from build123d import *

# Parameters (mm, degrees)
BOSS_EXTRUDE1_DEPTH  = 3.175
M3_CLEARANCE_HOLE1_D = 3.2
SKETCH4_R            = 2.1336
CUT_EXTRUDE1_DEPTH   = 74.133031325
SKETCH5_W            = 3
SKETCH5_H            = 19.05
CUT_EXTRUDE2_DEPTH   = 74.133031325


with BuildPart() as part:
    # Sketch1 → Boss-Extrude1 (new body)
    with BuildSketch(Plane(origin=(0, 0, 0), x_dir=(1, 0, 0), z_dir=(0, 1, 0))):
        Polygon((0, 0), (19.05, 0), (19.05, -3.175), (38.1, -3.175), (38.1, 0), (51.435, 0), (51.435, 7.62), (46.6725, 7.62), (46.6725, 15.24), (51.435, 15.24), (51.435, 22.86), (46.6725, 22.86), (46.6725, 30.48), (51.435, 30.48), (51.435, 51.8922), (0, 51.8922), align=None)
    extrude(amount=BOSS_EXTRUDE1_DEPTH)

    # M3 Clearance Hole1 (through all)
    with Locations(Plane(origin=(0, 3.175, 0), x_dir=(1, 0, 0), z_dir=(0, 1, 0))):
        with Locations((48.26, 19.05)):
            Hole(M3_CLEARANCE_HOLE1_D / 2)

    # Sketch4 → Cut-Extrude1 (cut, through all)
    with BuildSketch(Plane(origin=(0, 3.175, 0), x_dir=(1, 0, 0), z_dir=(0, 1, 0))):
        with Locations(Location((28.575, 27.305, 0), (0, 0, 270))):
            Circle(SKETCH4_R)
    extrude(amount=-CUT_EXTRUDE1_DEPTH, mode=Mode.SUBTRACT)

    # Sketch5 → Cut-Extrude2 (cut, through all)
    with BuildSketch(Plane(origin=(0, 3.175, 0), x_dir=(1, 0, 0), z_dir=(0, 1, 0))):
        with Locations((4.215, 19.05)):
            Rectangle(SKETCH5_W, SKETCH5_H)
    extrude(amount=-CUT_EXTRUDE2_DEPTH, mode=Mode.SUBTRACT)


solid = part.part
Check sheet for the modelled part. Datum: model origin and axes. Units: mm. A direction names the side the tool comes from. Round coordinates to 2 decimals unless told otherwise and drop trailing zeros. Order: outer loops, then holes, each group sorted by start corner. A loop starts at its lowest first (then second) coordinate and runs counter-clockwise, first axis right, second up.
Q1. Scan lines: L1, parallel to X at y = 1.25, z = -19.05 (3 decimals); L2, parallel to X at y = 1.65, z = -11 (1 decimal); L3, parallel to Z at x = 28.5, y = 1 (3 decimals). Record each from-to range of solid material in increasing order.
Filled sheet:
L1: x = 0 to 2.715, 5.715 to 46.66, 49.86 to 51.435
L2: x = 0 to 2.7, 5.7 to 46.7
L3: z = -51.892 to -29.437, -25.173 to 3.175
Q2. Cross-section at D-D, the plane x = 39.5. Enter the section's corners in (y, z) (3 decimals), plus the area to 3 significant figures.
Filled sheet:
outline: (0, -51.892) - (3.175, -51.892) - (3.175, 0) - (0, 0) - close
area: 165 mm2
Q3. Set-up check for faces 5 (the face through (5.715, 2, -19)), 6 (the face through (49, 2, -15.24)), 7 (the face through (38.1, 2, 2)): record each of +Z, -Z, +X, -X, +Y, -Y from which the full face is reachable in a straight line by a thin tool's end or side.
Filled sheet:
face 5: +Y, -Y
face 6: +X, +Y, -Y
face 7: +Z, +X, +Y, -Y
Q4. Depth check by flat-ended pin: P1, Ø3, axis at x = 12.5, z = -7.5, coming from the -Y side; P2, Ø1, axis at x = 49, y = 1.5, coming from the +Z side; P3, Ø1, axis at y = 2, z = -14.5, coming from the +X side. Enter the tip coordinate at first touch or a pass-through.
Filled sheet:
P1: stops at y = 0
P2: stops at z = 0
P3: stops at x = 46.67
Q5. Cross-section at B-B, the plane x = 48.26. Enter the section's corners in (y, z) (3 decimals).
Filled sheet:
outline: (0, -51.892) - (3.175, -51.892) - (3.175, -30.48) - (0, -30.48) - close; (0, -22.86) - (3.175, -22.86) - (3.175, -20.65) - (0, -20.65) - close; (0, -17.45) - (3.175, -17.45) - (3.175, -15.24) - (0, -15.24) - close; (0, -7.62) - (3.175, -7.62) - (3.175, 0) - (0, 0) - close
Q6. Draft check along Z on faces 1 (the face through (4, 2, -28.575)), 2 (the face through (4, 2, -9.525)), 3 (the face through (51.435, 2, -19)), 4 (the face through (9, 2, 0)). Enter one of: pulls with the +Z half, pulls with the -Z half, needs draft (parallel to the pull), parting line crosses it, or undercut.
Filled sheet:
face 1: undercut
face 2: undercut
face 3: needs draft
face 4: pulls with the +Z half
Q7. Cross-section at A-A, the plane z = -14.5. Enter the section's corners in (x, y) (1 decimal).
Filled sheet:
outline: (0, 0) - (2.7, 0) - (2.7, 3.2) - (0, 3.2) - close; (5.7, 0) - (46.7, 0) - (46.7, 3.2) - (5.7, 3.2) - close
Q8. Cross-section at C-C, the plane y = 2.55. Give the number of separate pieces and of enclosed holes in the cut face, plus the area to 3 significant figures.
Filled sheet:
separate pieces: 1
enclosed holes: 3
area: 2,580 mm2
